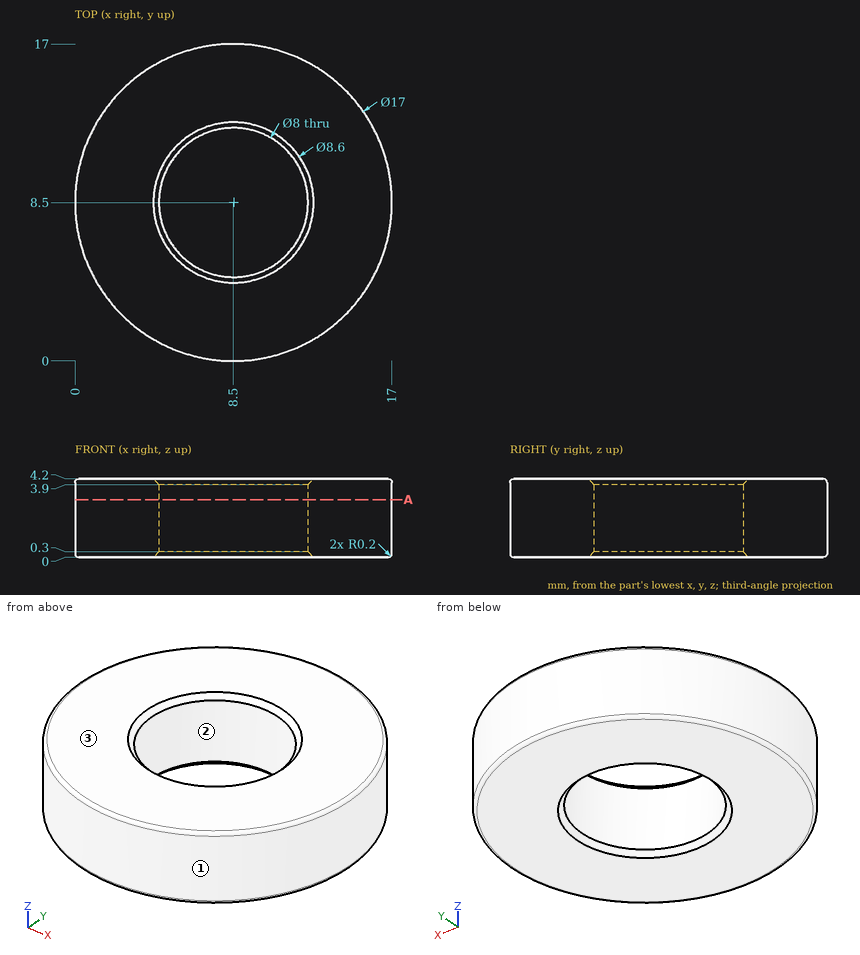
Answer from the drawing. Dimensions are ordinates in mm from the lowest x, y and z of the part. Coordinates: 2 decimals unless noted, no trailing zeros. Write each loop counter-clockwise with the first axis right and the second up, starting at its lowest first coordinate (ties: lowest second). Pieces come first, ordered by that corner, then holes. Notation, with made-up numbers: M -7,23 L 18,23 A34 ccw 18,60 Z; hole C 65,-5.5 d10. An arc over 180 degrees is marked long. Write item = value, one per line.
1. Determine the mould class of the marked faces 1, 2 and 3 for opening direction Y: released by +Y, released by -Y, zero draft, split by the parting line, or undercut.
Solution:
face_1 = split by the parting line
face_2 = undercut
face_3 = zero draft
2. The part is cut by section A-A (z = 3.1). Determine the outline of the cut face in (x, y).
Solution:
outline = C 8.5,8.5 d17; hole C 8.5,8.5 d8
3. Straight lines are drawn through the part: line 1 (Y direction, x = 8.5, z = 1); line 2 (Y direction, x = 6.75, z = 3.65); line 3 (X direction, y = 11.75, z = 1.4). For each, find the intervals that lie inside material, in ascending order. Write a range as from..to.
Solution:
line_1 = 0..4.5, 12.5..17
line_2 = 0.18..4.9, 12.1..16.82
line_3 = 0.65..6.17, 10.83..16.35
4. Flat-ended cylindrical pins translate along their axes: pin 1 (1 mm diameter, centred on x = 5.5, z = 3.5, fed in from +Y); pin 2 (1 mm diameter, centred on y = 4.5, z = 3, fed in from -X); pin 3 (1 mm diameter, centred on x = 3, z = 2.5, fed in from -Y); pin 4 (6.5 mm diameter, centred on x = 8.5, y = 8.5, fed in from -Z). Find the tip coordinate at first contact, or state that the pin passes through.
Solution:
pin_1 = 16.62
pin_2 = 0.75
pin_3 = 1.63
pin_4 = through
